Answer from the drawing. Dimensions are ordinates in mm from the lowest x, y and z of the part. A direction names the side the tool comes from. Round coordinates to 2 decimals unless told otherwise and drop trailing zeros. Order: outer loops, then holes, each group sorted by start corner. A loop starts at its lowest first (then second) coordinate and runs counter-clockwise, first axis right, second up. Notation, with made-up numbers: (-19.5, 28) -> (-9.5, 28) arc R14 ccw to (-9.5, 38) -> close; hole circle Ø8 at (56, 77.5). An arc over 180 degrees is marked (long way). Use a Markdown table: item, result. Add a question column.
1. Consider L1, parallel to Y at x = 15, z = 4.25 (1 decimal); L2, parallel to Y at x = 13, z = 5.75 (1 decimal); L3, parallel to Z at x = 6.25, y = 4.75. Determine where each line is inside the solid, lowest interval first. Write a range as [from, to].
2. Section C-C, the plane z = 14 is taken. Give the vertices of the cut face in (x, y) (1 decimal).
3. Section D-D, the plane y = 2 is taken. Give the vertices of the cut face in (x, z) (1 decimal).
4. For the marked faces 4, 5 and 6, determine the directions among +Z, -Z, +X, -X, +Y, -Y from which every point of the face is accessible in a straight line to the end or side of a thin tool.
5. The mould has two halves that part along X. Classify the marked faces 1, 2 and 3: +X half, -X half, draft (parallel to the pull), parting line (faces both ways), or undercut.
6. Section B-B, the plane x = 3.5 is taken. Give the vertices of the cut face in (y, z) (1 decimal), then the cut area to 3 significant figures.
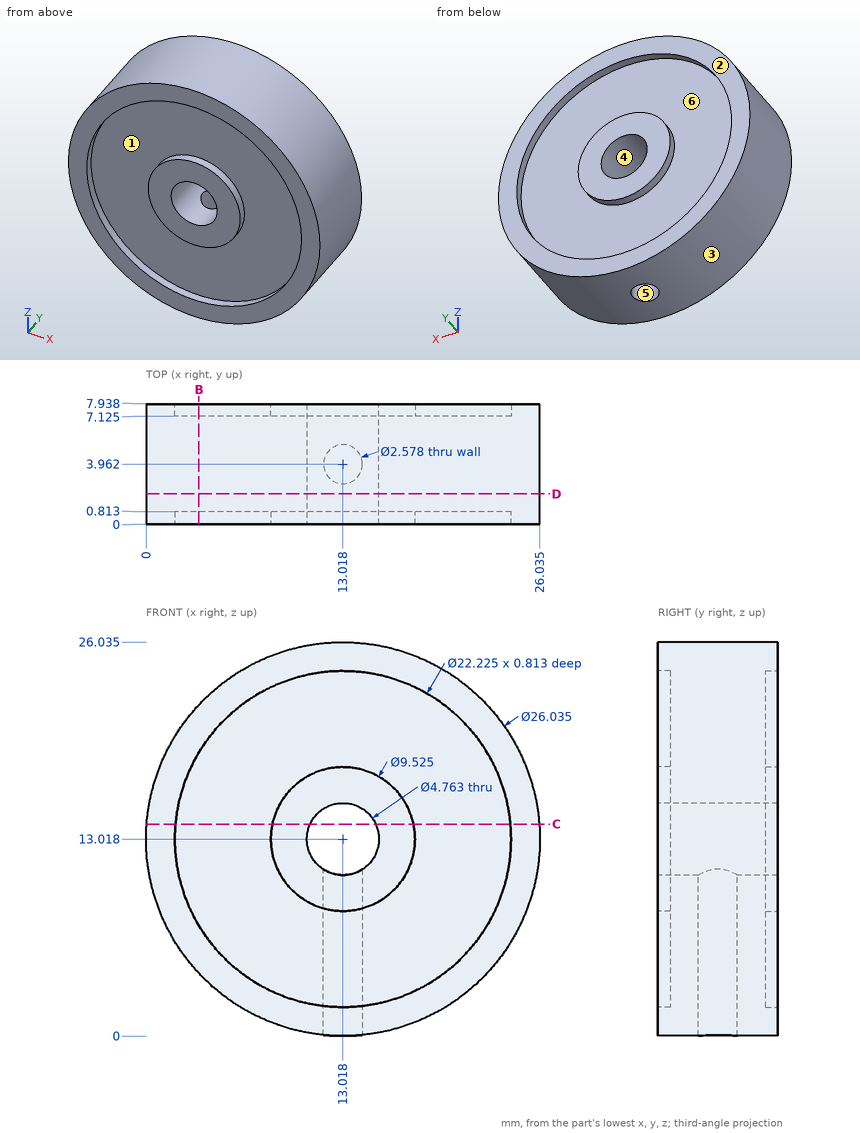
Verdict:
| question | item | result |
|---|---|---|
| 1 | L1 | y = [0.8, 7.1] |
| 1 | L2 | y = [0.8, 2.7], [5.3, 7.1] |
| 1 | L3 | z = [1.9, 24.14] |
| 2 | outline | (0, 0) -> (1.9, 0) -> (1.9, 0.8) -> (8.4, 0.8) -> (8.4, 0) -> (10.8, 0) -> (10.8, 7.9) -> (8.4, 7.9) -> (8.4, 7.1) -> (1.9, 7.1) -> (1.9, 7.9) -> (0, 7.9) -> close; (15.2, 0) -> (17.7, 0) -> (17.7, 0.8) -> (24.1, 0.8) -> (24.1, 0) -> (26, 0) -> (26, 7.9) -> (24.1, 7.9) -> (24.1, 7.1) -> (17.7, 7.1) -> (17.7, 7.9) -> (15.2, 7.9) -> close |
| 3 | outline | circle Ø26 at (13, 13); hole circle Ø4.8 at (13, 13) |
| 4 | face 4 | +Y, -Y |
| 4 | face 5 | -Z |
| 4 | face 6 | +Y |
| 5 | face 1 | undercut |
| 5 | face 2 | draft |
| 5 | face 3 | parting line |
| 6 | outline | (0, 4.1) -> (7.9, 4.1) -> (7.9, 7.3) -> (7.1, 7.3) -> (7.1, 18.8) -> (7.9, 18.8) -> (7.9, 21.9) -> (0, 21.9) -> (0, 18.8) -> (0.8, 18.8) -> (0.8, 7.3) -> (0, 7.3) -> close |
| 6 | area | 122 mm2 |
